Read the model definition and answer for the solid it produces. Units are mm, in the model's axes. Face numbers are marked on the shaded views. A direction names the side the tool comes from. Coordinates: 2 decimals unless noted, no trailing zeros. Write each loop counter-clockwise with the first axis right and the second up, starting at its lowest first coordinate (ties: lowest second). Pieces come first, ordered by that corner, then holes.
Item 1: A tool of negligible diameter and unlimited length cuts with its end or side. For the marked faces 1, 2 and 3, from which of +Z, -Z, +X, -X, +Y, -Y can it reach the whole face along a straight path? Write none if from no direction.
Item 2: Straight lines are drawn through the part: probe 1 along X at (y, z) = (-9, -70.5); probe 2 along X at (y, z) = (-4, -53.5); probe 3 along Z at (x, y) = (12, -7.5). For each, find the intervals that lie inside material, in ascending order.
Item 3: Determine the mould class of the marked faces 4, 5 and 6 for opening direction Z: released by +Z, released by -Z, zero draft, split by the parting line, or undercut.
Item 4: Section C-C (x = -20) is taken. Give the vertices of the cut face in (y, z).
Item 5: Section B-B (z = -36.5) is taken. Give the vertices of the cut face in (x, y).
Item 6: Section D-D (x = 1) is taken. Give the vertices of the cut face in (y, z), then the cut area to 3 significant figures.
Item 7: Each of these flat-tipped pins is pushed along its axis until it touches: P1, Ø4, axis at x = 2.5, y = -6, coming from the +Z side; P2, Ø12, axis at y = -12.5, z = -63.5, coming from the +X side; P3, Ø14.5, axis at x = 14.5, y = -19.5, coming from the -Z side; P4, Ø3, axis at x = 26, z = -71.5, coming from the +Y side. Where does it stop, or does it pass through?
from build123d import *

# Parameters (mm, degrees)
PAD036_DEPTH = 6
PAD037_DEPTH = 6
PAD038_DEPTH = 12
PAD014_DEPTH = 20
PAD012_DEPTH = 33
PAD013_DEPTH = 20
PAD001_DEPTH = 33


with BuildPart() as pad036:
    # Sketch040 → Pad036 (new body)
    with BuildSketch(Plane.XZ.offset(4)):
        Polygon((-22.876627, -50.458862), (-2.795745, -40.418423), (3.522805, -28.90654), (-39.408733, -32.801537), align=None)
    extrude(amount=PAD036_DEPTH)


with BuildPart() as pad037:
    # Sketch041 → Pad037 (new body)
    with BuildSketch(Plane.XZ.offset(24)):
        Polygon((-22.876627, -50.458862), (-2.795745, -40.418423), (3.522805, -28.90654), (-39.408733, -32.801537), align=None)
    extrude(amount=PAD037_DEPTH)


with BuildPart() as pad038:
    # Sketch042 → Pad038 (new body)
    with BuildSketch(Plane.XZ.offset(8)):
        Polygon((26.854265, -42.508881), (4.226509, -42.508881), (-12.077076, -26.263317), (32.65625, -19.126871), align=None)
    extrude(amount=PAD038_DEPTH)


with BuildPart() as pad014:
    # Sketch018 → Pad014 (new body)
    with BuildSketch(Plane(origin=(10, -7, 0), x_dir=(1, 0, 0), z_dir=(0, -1, 0))):
        Polygon((12.921668, -76.043343), (12.921668, -72.681298), (10.907037, -71.064545), (12.949577, -67.987406), (17.894252, -67.987406), (19.953335, -71.012405), (17.993304, -72.648705), (17.981073, -76.043343), align=None)
    extrude(amount=PAD014_DEPTH)


with BuildPart() as pad012:
    # Sketch016 → Pad012 (new body)
    with BuildSketch(Plane.XZ):
        Polygon((31.922119, -73.764191), (34.715668, -84.347412), (31.00419, -84.347412), (29.994871, -83.010223), (29.004835, -82.997353), (29.97435, -84.356453), (27.001257, -84.356453), (25.99424, -83.013763), (24.977634, -83.013763), (26.003832, -84.375633), (23.007538, -84.375633), (22.019703, -83.023636), (20.974325, -83.023636), (22.000523, -84.366325), (19.017838, -84.366325), (17.99164, -83.004456), (16.984625, -83.004456), (18.00123, -84.366325), (15.032244, -84.366325), (14.013124, -83.020378), (12.982291, -83.020378), (14.00141, -84.379204), (12.681671, -84.379204), (4.650895, -73.764191), align=None)
    extrude(amount=PAD012_DEPTH)


with BuildPart() as fusion:
    # Sketch017 → Pad013 (new body)
    with BuildSketch(Plane(origin=(-4, -7, 0), x_dir=(1, 0, 0), z_dir=(0, -1, 0))):
        Polygon((12.921668, -76.043343), (12.921668, -72.681298), (10.907037, -71.064545), (12.949577, -67.987406), (17.894252, -67.987406), (19.953335, -71.012405), (17.993304, -72.648705), (17.981073, -76.043343), align=None)
    extrude(amount=PAD013_DEPTH)

    # Fusion001: union Pad012
    add(pad012.part)

    # Fusion: union Pad014
    add(pad014.part)


with BuildPart() as cut009:
    # Sketch001 → Pad001 (new body)
    with BuildSketch(Plane(origin=(-15, 0, -10), x_dir=(0.819152, 0, 0.573576), z_dir=(0, -1, 0))):
        Polygon((-26.184557, -19.824878), (-21.536683, -15.979609), (13.963177, -33.561758), (16.497322, -39.355457), (1.912507, -79.157962), (-20.506964, -63.527428), align=None)
    extrude(amount=PAD001_DEPTH)

    # Cut: cut Fusion
    add(fusion.part, mode=Mode.SUBTRACT)

    # Cut007: cut Pad038
    add(pad038.part, mode=Mode.SUBTRACT)

    # Cut008: cut Pad037
    add(pad037.part, mode=Mode.SUBTRACT)

    # Cut009: cut Pad036
    add(pad036.part, mode=Mode.SUBTRACT)


solid = cut009.part
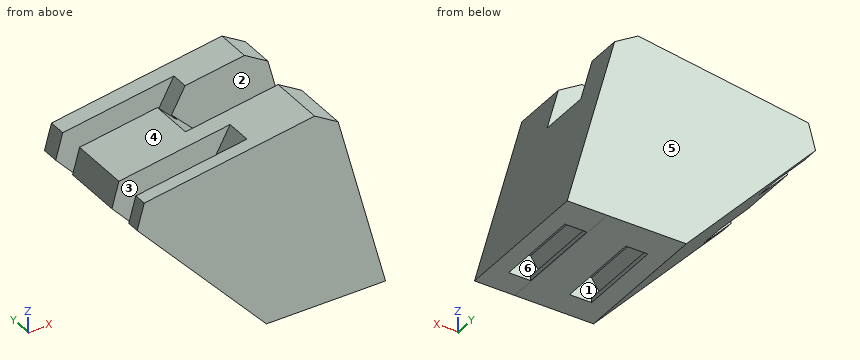
Established:
1. face 1: none
1. face 2: +Z, +X
1. face 3: +Z, -X
2. probe 1: x = 1.63 to 7.28, 15.6 to 21.28, 29.6 to 31.11
2. probe 2: x = -13.9 to 26.59
2. probe 3: z = -67.99 to -30.04
3. face 4: released by +Z
3. face 5: zero draft
3. face 6: undercut
4. outline: (-33, -46.82) - (-30, -46.82) - (-30, -34.91) - (-33, -34.91) - close; (-24, -46.82) - (-10, -46.82) - (-10, -34.91) - (-24, -34.91) - close; (-4, -46.82) - (0, -46.82) - (0, -34.91) - (-4, -34.91) - close
5. outline: (-23.77, -33) - (22.08, -33) - (22.08, -20) - (-1.8, -20) - (-1.8, -10) - (-23.77, -10) - (-23.77, -24) - (-0.65, -24) - (-0.65, -30) - (-23.77, -30) - close; (-23.77, -4) - (-0.65, -4) - (-0.65, -8) - (22.08, -8) - (22.08, 0) - (-23.77, 0) - close
6. outline: (-33, -69.82) - (0, -69.82) - (0, -31.72) - (-4, -31.72) - (-4, -33.5) - (-8, -33.5) - (-8, -39.29) - (-20, -39.29) - (-20, -31.72) - (-24, -31.72) - (-24, -33.5) - (-30, -33.5) - (-30, -31.72) - (-33, -31.72) - close
6. area: 1,150 mm2
7. P1: stops at z = -31.19
7. P2: stops at x = 30.84
7. P3: stops at z = -73.76
7. P4: stops at y = 0
